```python
from build123d import *

# Parameters (mm, degrees)
CROQUIS3_W              = 4
CROQUIS3_H              = 7.21110255
SALIENTE_EXTRUIR1_DEPTH = 15
CHAFL_N1_SIZE           = 1


with BuildPart() as part:
    # Croquis2 → Revolución1 (revolve)
    with BuildSketch(Plane.XY):
        Polygon((-4.25, 30), (-14.725, 30), (-15.725, 29), (-15.725, 1), (-14.725, 0), (-13.725, 0), (-12.725, 1), (-12.725, 14), (-11.725, 15), (-4.25, 15), align=None)
    revolve(axis=Axis((0, 0, 0), (0, 1, 0)))

    # Croquis3 → Saliente-Extruir1 (add)
    with BuildSketch(Plane(origin=(0, 30, 0), x_dir=(1, 0, 0), z_dir=(0, 1, 0))):
        with Locations((-4.25, 0)):
            Rectangle(CROQUIS3_W, CROQUIS3_H)
    extrude(amount=-SALIENTE_EXTRUIR1_DEPTH)

    # Chaflán1
    chafl_n1_edges = [part.edges().sort_by_distance(p)[0] for p in [
        (4.25, 30, 0),
        (-2.25, 30, 0),
    ]]
    chamfer(chafl_n1_edges, length=CHAFL_N1_SIZE)


solid = part.part
```
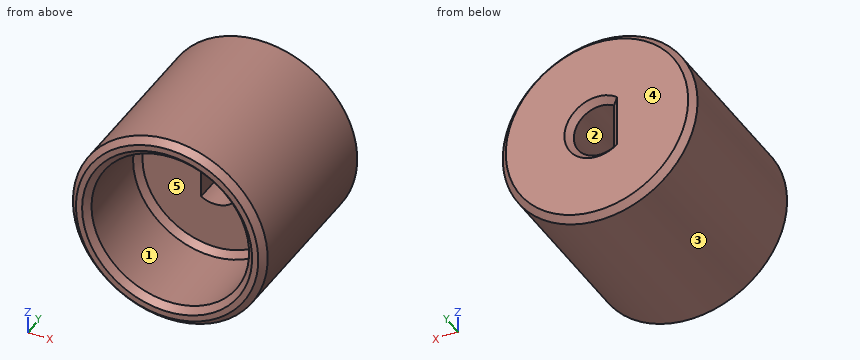
The listing builds one solid part. Answer for the finished solid, in the listing's coordinates (mm). Face numbers are marked on the shaded views. A direction names the side the tool comes from. Give positions to 0.01 mm unless a question says otherwise; leave off trailing zeros. Order: outer loops, then holes, each group sorted by start corner. A loop starts at its lowest first (then second) coordinate and runs counter-clockwise, first axis right, second up.
1) Find section B-B on x = 0. Write down the section's boundary in (y, z) (3 decimals).
Reported:
outline: (0, -14.725) - (1, -15.725) - (29, -15.725) - (30, -14.725) - (30, -5.25) - (29, -4.25) - (15, -4.25) - (15, -11.725) - (14, -12.725) - (1, -12.725) - (0, -13.725) - close; (0, 13.725) - (1, 12.725) - (14, 12.725) - (15, 11.725) - (15, 4.25) - (29, 4.25) - (30, 5.25) - (30, 14.725) - (29, 15.725) - (1, 15.725) - (0, 14.725) - close
2) Find section D-D on y = 26. Write down the section's boundary in (x, z) (3 decimals), then the cut area to 3 significant figures.
Reported:
outline: circle Ø31.45 at (0, 0); hole (-2.25, -3.606) arc R4.25 ccw (long way) to (-2.25, 3.606) - close
area: 730 mm2
3) Consider line 1 along Z through (x, y) = (0, 25.25) (3 decimals); line 2 along Z through (x, y) = (1, 18); line 3 along Y through (x, z) = (4, -4). Determine where each line is inside the solid, lowest interval first.
Reported:
line 1: z = -15.725 to -4.25, 4.25 to 15.725
line 2: z = -15.69 to -4.13, 4.13 to 15.69
line 3: y = 15 to 30
4) Determine the mould class of the marked faces 3, 4 and 5 for opening direction X: pulls with the +X half, pulls with the -X half, needs draft (parallel to the pull), parting line crosses it, or undercut.
Reported:
face 3: parting line crosses it
face 4: needs draft
face 5: undercut
5) Given P1, Ø10, axis at x = -1, z = -8, coming from the -Y side; P2, Ø3, axis at x = 8, y = 20.5, coming from the +Z side; P3, Ø1.5, axis at y = 17, z = 5, coming from the +X side, each flat-ended and moving along its own axis, determine where each tip first touches the part or whether it passes through.
Reported:
P1: stops at y = 0.66
P2: stops at z = 14.32
P3: stops at x = 15.14
6) Find section A-A on z = 0. Write down the section's boundary in (x, y) (3 decimals), then the cut area to 3 significant figures.
Reported:
outline: (-15.725, 1) - (-14.725, 0) - (-13.725, 0) - (-12.725, 1) - (-12.725, 14) - (-11.725, 15) - (-2.25, 15) - (-2.25, 29) - (-3.25, 30) - (-14.725, 30) - (-15.725, 29) - close; (4.25, 15) - (11.725, 15) - (12.725, 14) - (12.725, 1) - (13.725, 0) - (14.725, 0) - (15.725, 1) - (15.725, 29) - (14.725, 30) - (5.25, 30) - (4.25, 29) - close
area: 461 mm2
7) For the marked faces 1 and 2, determine the directions among +Z, -Z, +X, -X, +Y, -Y from which every point of the face is accessible in a straight line to the end or side of a thin tool.
Reported:
face 1: -Y
face 2: +Y, -Y
8) Find section C-C on y = 11.5. Write down the section's boundary in (x, z) (3 decimals).
Reported:
outline: circle Ø31.45 at (0, 0); hole circle Ø25.45 at (0, 0)
